Check sheet for the modelled part. Datum: model origin and axes. Units: mm. A direction names the side the tool comes from. Coordinates: 2 decimals unless noted, no trailing zeros. Loops run counter-clockwise (first coordinate to the right, second up) from the corner with the lowest first, then second, coordinate; pieces in that order, holes last. Notation, with made-up numbers: (50, -37.5) -> (88, -37.5) arc R24 ccw to (88, -22.5) -> close; hole circle Ø2 at (81.5, -22). An arc over 180 degrees is marked (long way). Use one line per item in the form item = value.
from build123d import *

# Parameters (mm, degrees)
F0_R     = 10
F1_DEPTH = 2
F2_R     = 15
F3_DEPTH = 2
F4_R     = 2.5
F5_DEPTH = 12


with BuildPart() as f1:
    # F0 (on Top) → F1 (new body)
    with BuildSketch(Plane.XY):
        Circle(F0_R)
    extrude(amount=F1_DEPTH)

    # F2 (on face) → F3 (join)
    with BuildSketch(Plane.XY.offset(2)):
        Circle(F2_R)
    extrude(amount=F3_DEPTH)

    # F4 (on face) → F5 (join)
    with BuildSketch(Plane.XY.offset(4)):
        with Locations((-5, 0)):
            Circle(F4_R)
        with Locations((5, 0)):
            Circle(F4_R)
    extrude(amount=F5_DEPTH)


solid = f1.part
(1) Mould release check, pull along X, two halves, no side actions. Record for faces 4 (the cylindrical face through (-14.985, 0.66, 2.986)), 5 (the flat face through (5, 0, 16)), 6 (the cylindrical face through (-2.615, 0.751, 9.916)): +X half, -X half, draft (parallel to the pull), parting line (faces both ways), or undercut.
Established:
face_4 = parting line
face_5 = draft
face_6 = undercut
(2) Section check B-B, the plane x = 0. Record the boundary of the cut face in (y, z), plus the area to 3 significant figures.
Established:
outline = (-15, 2) -> (-10, 2) -> (-10, 0) -> (10, 0) -> (10, 2) -> (15, 2) -> (15, 4) -> (-15, 4) -> close
area = 100 mm²
(3) Section check C-C, the plane z = 2.75. Record the boundary of the cut face in (x, y), plus the area to 3 significant figures.
Established:
outline = circle Ø30 at (0, 0)
area = 707 mm²
(4) Section check D-D, the plane x = 5. Record the boundary of the cut face in (y, z), plus the area to 3 significant figures.
Established:
outline = (-14.14, 2) -> (-8.66, 2) -> (-8.66, 0) -> (8.66, 0) -> (8.66, 2) -> (14.14, 2) -> (14.14, 4) -> (2.5, 4) -> (2.5, 16) -> (-2.5, 16) -> (-2.5, 4) -> (-14.14, 4) -> close
area = 151 mm²
(5) Section check A-A, the plane y = 0. Record the boundary of the cut face in (x, z).
Established:
outline = (-15, 2) -> (-10, 2) -> (-10, 0) -> (10, 0) -> (10, 2) -> (15, 2) -> (15, 4) -> (7.5, 4) -> (7.5, 16) -> (2.5, 16) -> (2.5, 4) -> (-2.5, 4) -> (-2.5, 16) -> (-7.5, 16) -> (-7.5, 4) -> (-15, 4) -> close
(6) Tool access check on faces 1 (the cylindrical face through (7.385, 0.751, 9.916)), 2 (the flat face through (0, 0, 0)), 3 (the cylindrical face through (-2.17, -9.76, 0.99)). Record the directions out of +Z, -Z, +X, -X, +Y, -Y that give a thin tool (end or side, any length) a straight path to the whole face; none if there is none.
Established:
face_1 = +Z
face_2 = -Z, +X, -X, +Y, -Y
face_3 = -Z
(7) Go/stop test with flat-tipped pins: P1, Ø1.5, axis at x = -5.5, y = 9.5, coming from the +Z side; P2, Ø6, axis at x = 3, z = 4, coming from the -Y side. Record where each tip stops, or that it passes through.
Established:
P1 = 4
P2 = -15
(8) Scan lines: line 1 along Z through (x, y) = (10.25, 10); line 2 along Z through (x, y) = (0.25, 2); line 3 along Y through (x, z) = (4.25, 13.5). Record each from-to range of solid material in increasing order.
Established:
line_1 = 2 to 4
line_2 = 0 to 4
line_3 = -2.38 to 2.38
